```python
from build123d import *

# Parameters (mm, degrees)
SKETCH_1_W = 10
SKETCH_1_H = 10


with BuildPart() as part:
    # 扫描2: sweep along a path in 草图3
    with BuildLine(Plane(origin=(0, 0, 0), x_dir=(0, 0, -1), z_dir=(1, 0, 0))) as sweep_2_path:
        Line((5, 0), (5, 1400))
        Line((5, 1400), (47.426406871, 1442.426406871))
        Line((47.426406871, 1442.426406871), (147.426406871, 1442.426406871))
    # 草图1 → 扫描2 (sweep)
    with BuildSketch(Plane(origin=(0, 0, 0), x_dir=(1, 0, 0), z_dir=(0, 1, 0))):
        Rectangle(SKETCH_1_W, SKETCH_1_H)
    sweep(path=sweep_2_path.line, transition=Transition.RIGHT)


solid = part.part
```
Geometry check sheet. Reference: the model listing, model coordinates, mm. Coordinates: 2 decimals unless noted, no trailing zeros. Loops run counter-clockwise (first coordinate to the right, second up) from the corner with the lowest first, then second, coordinate; pieces in that order, holes last.
Item 1: Sectioned sample at B-B, the plane y = 593. Record the boundary of the cut face in (x, z).
Item 2: Go/stop test with flat-tipped pins: pin 1 Ø2 at (x, y) = (-3, 781.5) entering from -Z; pin 2 Ø1.5 at (x, z) = (2, -34) entering from +Y; pin 3 Ø4 at (x, z) = (-1.5, -38.5) entering from +Y. Record where each tip stops, or that it passes through.
Item 3: Thickness scan on line 1 (Z direction, x = -1.75, y = 488); line 2 (Y direction, x = 1.25, z = -49); line 3 (Y direction, x = 2.75, z = -30). Record the ranges inside material, lowest first.
Item 4: Sectioned sample at C-C, the plane z = -68. Record the boundary of the cut face in (x, y).
Item 5: Sectioned sample at A-A, the plane x = -0.75. Record the boundary of the cut face in (y, z).
Check result:
1. outline: (-5, -5) - (5, -5) - (5, 5) - (-5, 5) - close
2. pin 1: stops at z = -5
2. pin 2: stops at y = 1443.89
2. pin 3: stops at y = 1449.64
3. line 1: z = -5 to 5
3. line 2: y = 1442.43 to 1452.43
3. line 3: y = 1425 to 1439.14
4. outline: (-5, 1442.43) - (5, 1442.43) - (5, 1452.43) - (-5, 1452.43) - close
5. outline: (0, -5) - (1400, -5) - (1442.43, -47.43) - (1442.43, -147.43) - (1452.43, -147.43) - (1452.43, -43.28) - (1404.14, 5) - (0, 5) - close
